Input: dimensioned drawing with shaded views. Units: mm. Origin: part minimum x, y, z. A direction names the side the tool comes from. Give positions to 0.01 mm unless a question says otherwise; leave off trailing zeros. Write each loop counter-clockwise with the first axis right and the second up, starting at its lowest first coordinate (ties: lowest second). Pieces come first, ordered by that corner, then holes. Notation, with made-up numbers: (3, 80) -> (31, 80) arc R29 cw to (31, 103) -> close; hole circle Ø3 at (36, 57). An arc over 180 degrees is marked (long way). Return JSON: item names as keys, results as strings. Group by question number.
Item 1: Line query: line 1 (Z direction, x = 3.75, y = 3.45). Output: solid intervals per line, ascending. Write a range as [from, to].
Item 2: Section B-B, the plane z = 0.5. Return loops of the section in (x, y).
Item 3: Section D-D, the plane x = 6.25. Return loops of the section in (y, z).
Item 4: Pin query (flat end, axial travel): P1, Ø1.5, axis at x = 5.5, y = 2, coming from the +Z side. Return the tip coordinate at first contact, or that it passes through.
Item 5: Section A-A, the plane x = 2.5. Return loops of the section in (y, z).
Item 6: Mould query, pull axis X, two halves, no side actions, for the marked faces 3, 4, 5 and 6. Classes: released by +X, released by -X, zero draft, split by the parting line, or undercut.
Item 7: Set-up query: the marked faces 1 and 2. Return all of +Z, -Z, +X, -X, +Y, -Y with unobstructed straight access to the full face (end or side cutting, diameter ignored); none if empty.
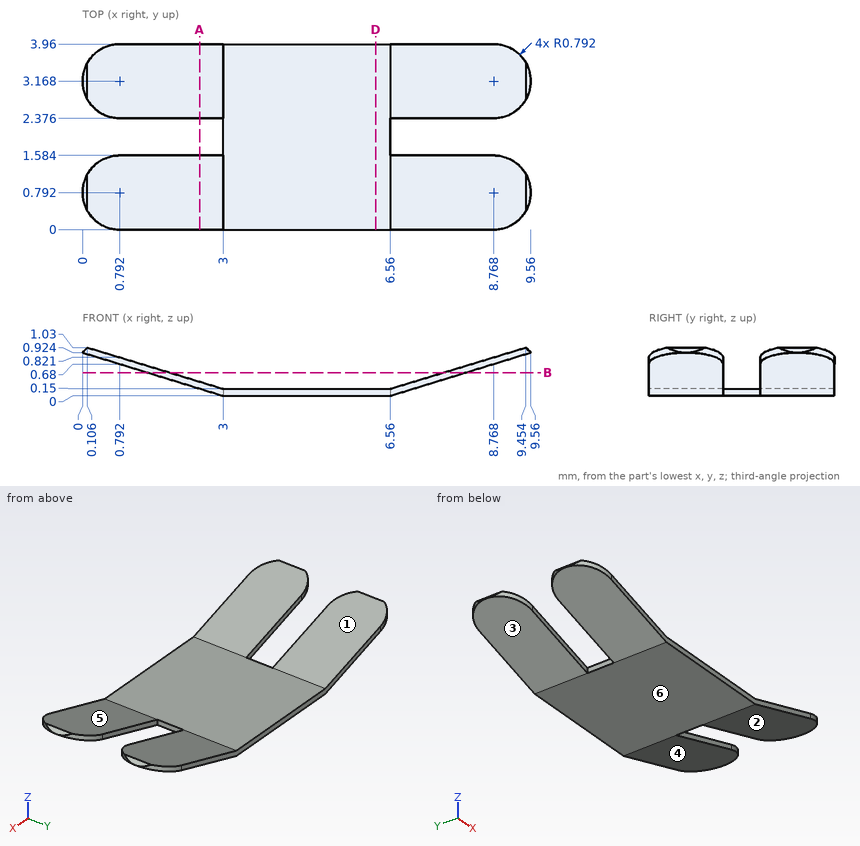
Answer below:
{
 "1": {"line 1": "z = [0, 0.15]"},
 "2": {"outline": "(1.38, 0) -> (1.85, 0) -> (1.85, 1.58) -> (1.38, 1.58) -> close; (1.38, 2.38) -> (1.85, 2.38) -> (1.85, 3.96) -> (1.38, 3.96) -> close; (7.71, 0) -> (8.18, 0) -> (8.18, 1.58) -> (7.71, 1.58) -> close; (7.71, 2.38) -> (8.18, 2.38) -> (8.18, 3.96) -> (7.71, 3.96) -> close"},
 "3": {"outline": "(0, 0) -> (3.96, 0) -> (3.96, 0.15) -> (0, 0.15) -> close"},
 "4": {"P1": "stops at z = 0.15"},
 "5": {"outline": "(0, 0.15) -> (1.58, 0.15) -> (1.58, 0.3) -> (0, 0.3) -> close; (2.38, 0.15) -> (3.96, 0.15) -> (3.96, 0.3) -> (2.38, 0.3) -> close"},
 "6": {"face 3": "released by -X", "face 4": "released by +X", "face 5": "undercut", "face 6": "zero draft"},
 "7": {"face 1": "+Z, +Y, -Y", "face 2": "-Z, +X, +Y, -Y"}
}
